Part print with two shaded views. Sizes in mm from the minimum x, y, z corner. A direction names the side the tool comes from. Round coordinates to 2 decimals unless told otherwise and drop trailing zeros. Write each loop counter-clockwise with the first axis right and the second up, starting at its lowest first coordinate (ties: lowest second). Pieces come first, ordered by that corner, then holes. Notation, with made-up numbers: (-5.75, -16) -> (11.25, -16) arc R30 ccw to (11.25, 22) -> close; hole circle Ø9 at (54.25, -40). An arc over 180 degrees is marked (long way). Return JSON: item names as keys, results as strings. Group by question number.
(1) Tool access for the marked faces 1, 2 and 3: list every direction of +Z, -Z, +X, -X, +Y, -Y with a clear straight run to the whole face (end or side of a thin tool).
(2) Saw through at D-D (y = 10.5). List the corners of the cut face in (x, z) (1 decimal).
(3) Saw through at C-C (z = 44). List the corners of the cut face in (x, y) (1 decimal).
(4) Drop flat-ended pins along their axis: pin 1 Ø10 at (x, y) = (29.5, 8) entering from +Z; pin 2 Ø6 at (y, z) = (24.5, 81) entering from -X; pin 3 Ø5 at (y, z) = (36, 37.5) entering from +X. Give the stop position or say it passes through.
(5) Saw through at B-B (y = 16). List the corners of the cut face in (x, z) (1 decimal).
(6) Drill centre lines: L1, parallel to Z at x = 21.5, y = 12; L2, parallel to Z at x = 23, y = 25; L3, parallel to X at y = 44.5, z = 25.5 (1 decimal). Where is each one in solid material? Low to high. Write a range as from..to.
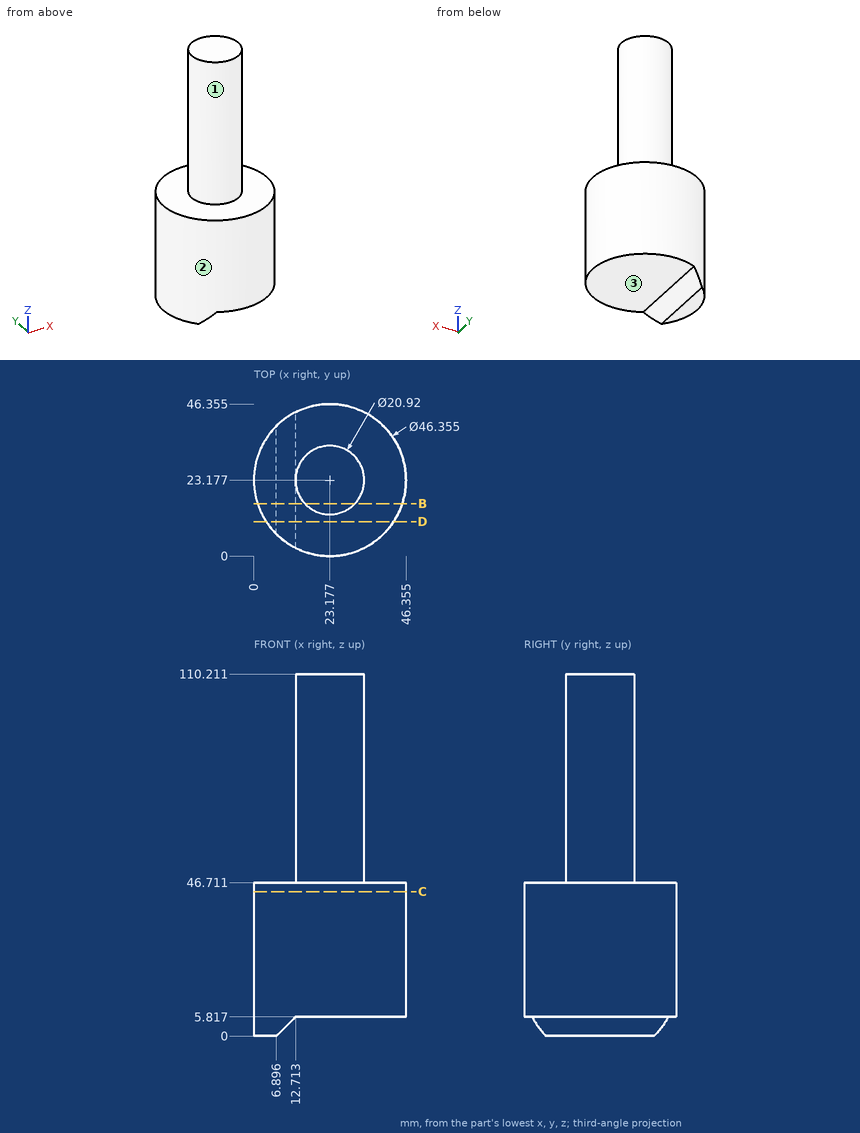
Computed values:
{
 "1": {"face 1": "+Z", "face 2": "+Z, -Z", "face 3": "-Z, +X, +Y, -Y"},
 "2": {"outline": "(3.8, 0) -> (6.9, 0) -> (12.7, 5.8) -> (42.6, 5.8) -> (42.6, 46.7) -> (3.8, 46.7) -> close"},
 "3": {"outline": "circle Ø46.4 at (23.2, 23.2)"},
 "4": {"pin 1": "z = 46.71", "pin 2": "x = 12.72", "pin 3": "x = 43.93"},
 "5": {"outline": "(1.1, 0) -> (6.9, 0) -> (12.7, 5.8) -> (45.2, 5.8) -> (45.2, 46.7) -> (30.8, 46.7) -> (30.8, 110.2) -> (15.6, 110.2) -> (15.6, 46.7) -> (1.1, 46.7) -> close"},
 "6": {"L1": "5.82..46.71", "L2": "5.82..110.21", "L3": "14.1..32.3"}
}
